from build123d import *

# Parameters (mm, degrees)
F1_DEPTH = 25


with BuildPart() as f1:
    # F0 (on Top) → F1 (new body)
    with BuildSketch(Plane.XY):
        with BuildLine():
            ThreePointArc((-31.476978, 49.874552), (-31.875369, 48.02339), (-33, 46.5))
            Line((-33, 46.5), (33, 46.5))
            ThreePointArc((33, 46.5), (31.605074, 48.808506), (31.780799, 51.5))
            Line((31.780799, 51.5), (-31.780799, 51.5))
            ThreePointArc((-31.780799, 51.5), (-31.553586, 50.701351), (-31.476978, 49.874552))
        make_face()
        with BuildLine():
            ThreePointArc((-38, 45.854927), (-35.401185, 45.411541), (-33, 46.5))
            ThreePointArc((-33, 46.5), (-31.875369, 48.02339), (-31.476978, 49.874552))
            ThreePointArc((-31.476978, 49.874552), (-31.553586, 50.701351), (-31.780799, 51.5))
            Line((-31.780799, 51.5), (-38, 51.5))
            Line((-38, 51.5), (-38, 45.854927))
        make_face()
        with BuildLine():
            ThreePointArc((-31.780799, 51.5), (-39.00144, 53.206613), (-38, 45.854927))
            Line((-38, 45.854927), (-38, 51.5))
            Line((-38, 51.5), (-31.780799, 51.5))
        make_face()
        with BuildLine():
            Line((-33, -46.5), (-33, 46.5))
            ThreePointArc((-33, 46.5), (-35.401185, 45.411541), (-38, 45.854927))
            Line((-38, 45.854927), (-38, -45.854927))
            ThreePointArc((-38, -45.854927), (-35.401185, -45.411541), (-33, -46.5))
        make_face()
        with BuildLine():
            ThreePointArc((40.476978, 49.874552), (36.803778, 54.297944), (31.780799, 51.5))
            Line((31.780799, 51.5), (38, 51.5))
            Line((38, 51.5), (38, 45.854927))
            ThreePointArc((38, 45.854927), (39.808009, 47.513789), (40.476978, 49.874552))
        make_face()
        with BuildLine():
            ThreePointArc((31.780799, 51.5), (31.605074, 48.808506), (33, 46.5))
            ThreePointArc((33, 46.5), (35.401185, 45.411541), (38, 45.854927))
            Line((38, 45.854927), (38, 51.5))
            Line((38, 51.5), (31.780799, 51.5))
        make_face()
        with BuildLine():
            ThreePointArc((38, 45.854927), (35.401185, 45.411541), (33, 46.5))
            Line((33, 46.5), (33, -46.5))
            ThreePointArc((33, -46.5), (35.401185, -45.411541), (38, -45.854927))
            Line((38, -45.854927), (38, 45.854927))
        make_face()
        with BuildLine():
            ThreePointArc((40.476978, -49.874552), (39.808009, -47.513789), (38, -45.854927))
            Line((38, -45.854927), (38, -51.5))
            Line((38, -51.5), (31.780799, -51.5))
            ThreePointArc((31.780799, -51.5), (36.803778, -54.297944), (40.476978, -49.874552))
        make_face()
        with BuildLine():
            ThreePointArc((38, -45.854927), (35.401185, -45.411541), (33, -46.5))
            ThreePointArc((33, -46.5), (31.605074, -48.808506), (31.780799, -51.5))
            Line((31.780799, -51.5), (38, -51.5))
            Line((38, -51.5), (38, -45.854927))
        make_face()
        with BuildLine():
            Line((33, -46.5), (-33, -46.5))
            ThreePointArc((-33, -46.5), (-31.875369, -48.02339), (-31.476978, -49.874552))
            ThreePointArc((-31.476978, -49.874552), (-31.553586, -50.701351), (-31.780799, -51.5))
            Line((-31.780799, -51.5), (31.780799, -51.5))
            ThreePointArc((31.780799, -51.5), (31.605074, -48.808506), (33, -46.5))
        make_face()
        with BuildLine():
            ThreePointArc((-31.476978, -49.874552), (-31.875369, -48.02339), (-33, -46.5))
            ThreePointArc((-33, -46.5), (-35.401185, -45.411541), (-38, -45.854927))
            Line((-38, -45.854927), (-38, -51.5))
            Line((-38, -51.5), (-31.780799, -51.5))
            ThreePointArc((-31.780799, -51.5), (-31.553586, -50.701351), (-31.476978, -49.874552))
        make_face()
        with BuildLine():
            Line((-38, -51.5), (-38, -45.854927))
            ThreePointArc((-38, -45.854927), (-39.00144, -53.206613), (-31.780799, -51.5))
            Line((-31.780799, -51.5), (-38, -51.5))
        make_face()
    extrude(amount=F1_DEPTH)


solid = f1.part
The model under review builds one solid part; all positions refer to its coordinate system, in mm. A direction names the side the tool comes from. Round coordinates to 2 decimals unless told otherwise and drop trailing zeros. Write each loop counter-clockwise with the first axis right and the second up, starting at its lowest first coordinate (ties: lowest second). Pieces come first, ordered by that corner, then holes. Notation, with made-up numbers: M 41.25,53 L 86.25,53 A33 cw 86.25,86 Z; hole C -23,-35 d3. An arc over 180 degrees is marked long. Use a Markdown table: item, result. Add a question column.
Q1. Machinability: for faces 1 (the face through (-38, 1, 12)), 2 (the face through (38, -1, 12)), 3 (the face through (0, 46.5, 12)), 4 (the face through (-37, 1, 25)), 5 (the face through (0, 51.5, 12)), which of the approach directions +Z, -Z, +X, -X, +Y, -Y give a long, thin tool a straight path to every point of the face, cutting with its end or side? Answer none if there is none.
Q2. We need section B-B, the plane z = 21. State the section outline as (x, y) points.
Q3. Insertion check: pin 1 (1 mm diameter, centred on y = 7, z = 5.5, fed in from -X); pin 2 (8 mm diameter, centred on x = -10, z = 4.5, fed in from +Y); pin 3 (7.5 mm diameter, centred on y = -10.5, z = 6.5, fed in from +X). Each pin has a flat end and moves straight along its axis. Give the tip position at first contact, or say it passes through.
Q4. We need section C-C, the plane y = -41. State the section outline as (x, z) points.
Q5. To check wall thickness, follow line 1 (Y direction, x = -3, z = 2); line 2 (X direction, y = 11, z = 20.25); line 3 (Y direction, x = 32, z = 9.5). State the ranges of each line that lie inside material, in increasing order.
Q6. The part is to be moulded in two halves that separate along Y. For faces 6 (the face through (33, 1, 12)), 7 (the face through (-37, 1, 0)), 8 (the face through (0, -51.5, 12)), say which applies: pulls with the +Y half, pulls with the -Y half, needs draft (parallel to the pull), parting line crosses it, or undercut.
Q7. We need section A-A, the plane x = -12. State the section outline as (y, z) points, plus the area to 3 significant figures.
Findings below:
| question | item | result |
|---|---|---|
| 1 | face 1 | +Z, -Z, -X |
| 1 | face 2 | +Z, -Z, +X |
| 1 | face 3 | +Z, -Z |
| 1 | face 4 | +Z, +X, -X, +Y, -Y |
| 1 | face 5 | +Z, -Z, +Y |
| 2 | outline | M -38,-45.85 A4.5 ccw long -31.78,-51.5 L 31.78,-51.5 A4.5 ccw long 38,-45.85 L 38,45.85 A4.5 ccw long 31.78,51.5 L -31.78,51.5 A4.5 ccw long -38,45.85 Z; hole M -33,-46.5 L 33,-46.5 L 33,46.5 L -33,46.5 Z |
| 3 | pin 1 | stops at x = -38 |
| 3 | pin 2 | stops at y = 51.5 |
| 3 | pin 3 | stops at x = 38 |
| 4 | outline | M -38,0 L -33,0 L -33,25 L -38,25 Z; M 33,0 L 38,0 L 38,25 L 33,25 Z |
| 5 | line 1 | y = -51.5 to -46.5, 46.5 to 51.5 |
| 5 | line 2 | x = -38 to -33, 33 to 38 |
| 5 | line 3 | y = -51.98 to -46.5, 46.5 to 51.98 |
| 6 | face 6 | undercut |
| 6 | face 7 | needs draft |
| 6 | face 8 | pulls with the -Y half |
| 7 | outline | M -51.5,0 L -46.5,0 L -46.5,25 L -51.5,25 Z; M 46.5,0 L 51.5,0 L 51.5,25 L 46.5,25 Z |
| 7 | area | 250 mm² |
